```python
from build123d import *

# Parameters (mm, degrees)
CROQUIS1_R              = 1.5
CROQUIS1_R_2            = 4
SALIENTE_EXTRUIR1_DEPTH = 6
CROQUIS4_R              = 4
SALIENTE_EXTRUIR3_DEPTH = 6
CORTAR_EXTRUIR1_DEPTH   = 6
REDONDEO3_R             = 4
CORTAR_EXTRUIR2_DEPTH   = 6
REDONDEO4_R             = 2.5
REDONDEO6_R             = 10


with BuildPart() as part:
    # Croquis1 → Saliente-Extruir1 (new body)
    with BuildSketch(Plane.XY):
        with BuildLine():
            Line((-17.112213819, 2.294275414), (-30.516043414, 23.123582692))
            ThreePointArc((-30.516043414, 23.123582692), (-31.14080226, 23.989156666), (-31.854269143, 24.783201331))
            Line((-31.854269143, 24.783201331), (-45.961940777, 38.890872965))
            Line((-45.961940777, 38.890872965), (-78.488852712, 71.4177849))
            Line((-78.488852712, 71.4177849), (-71.4177849, 78.488852712))
            Line((-71.4177849, 78.488852712), (-38.890872965, 45.961940777))
            Line((-38.890872965, 45.961940777), (-24.783201331, 31.854269143))
            ThreePointArc((-24.783201331, 31.854269143), (-23.989156666, 31.14080226), (-23.123582692, 30.516043414))
            Line((-23.123582692, 30.516043414), (-2.294275414, 17.112213819))
            ThreePointArc((-2.294275414, 17.112213819), (-0.610887166, 15.302496804), (0, 12.907567049))
            Line((0, 12.907567049), (0, 7.055686841))
            ThreePointArc((0, 7.055686841), (-0.823113423, 5.438609853), (-2.614937985, 5.15257064))
            Line((-2.614937985, 5.15257064), (-4.503911831, 5.762938925))
            ThreePointArc((-4.503911831, 5.762938925), (-5.518487605, 5.518487605), (-5.762938925, 4.503911831))
            Line((-5.762938925, 4.503911831), (-5.15257064, 2.614937985))
            ThreePointArc((-5.15257064, 2.614937985), (-5.438609853, 0.823113423), (-7.055686841, 0))
            Line((-7.055686841, 0), (-12.907567049, 0))
            ThreePointArc((-12.907567049, 0), (-15.302496804, 0.610887166), (-17.112213819, 2.294275414))
        make_face()
        with Locations((-38.890872965, 38.890872965)):
            Circle(CROQUIS1_R, mode=Mode.SUBTRACT)
        with Locations((-24.04163056, 24.04163056)):
            Circle(CROQUIS1_R, mode=Mode.SUBTRACT)
        with Locations((-15.25, 15.25)):
            Circle(CROQUIS1_R_2, mode=Mode.SUBTRACT)
    extrude(amount=SALIENTE_EXTRUIR1_DEPTH)

    # Croquis4 → Saliente-Extruir3 (add)
    with BuildSketch(Plane.XY.offset(6)):
        Polygon((-78.488852712, 71.4177849), (-89.802561211, 71.4177849), (-103.944696834, 85.559920524), (-103.944696834, 103.944696834), (-85.559920524, 103.944696834), (-71.4177849, 89.802561211), (-71.4177849, 78.488852712), align=None)
        with Locations((-88.388347648, 88.388347648)):
            Circle(CROQUIS4_R, mode=Mode.SUBTRACT)
    extrude(amount=-SALIENTE_EXTRUIR3_DEPTH)

    # Croquis5 → Cortar-Extruir1 (cut)
    with BuildSketch(Plane.XY.offset(6)):
        with BuildLine():
            Line((-99.348502757, 96.166522241), (-97.227182413, 94.045201898))
            ThreePointArc((-97.227182413, 94.045201898), (-94.045201898, 94.045201898), (-94.045201898, 97.227182413))
            Line((-94.045201898, 97.227182413), (-96.166522241, 99.348502757))
            ThreePointArc((-96.166522241, 99.348502757), (-99.348502757, 99.348502757), (-99.348502757, 96.166522241))
        make_face()
        with BuildLine():
            Line((-89.888347648, 80.638347648), (-89.888347648, 78.638347648))
            ThreePointArc((-89.888347648, 78.638347648), (-88.388347648, 77.138347648), (-86.888347648, 78.638347648))
            Line((-86.888347648, 78.638347648), (-86.888347648, 80.638347648))
            ThreePointArc((-86.888347648, 80.638347648), (-88.388347648, 82.138347648), (-89.888347648, 80.638347648))
        make_face()
        with BuildLine():
            Line((-80.638347648, 86.888347648), (-78.638347648, 86.888347648))
            ThreePointArc((-78.638347648, 86.888347648), (-77.138347648, 88.388347648), (-78.638347648, 89.888347648))
            Line((-78.638347648, 89.888347648), (-80.638347648, 89.888347648))
            ThreePointArc((-80.638347648, 89.888347648), (-82.138347648, 88.388347648), (-80.638347648, 86.888347648))
        make_face()
        with BuildLine():
            Line((-96.138347648, 89.888347648), (-98.138347648, 89.888347648))
            ThreePointArc((-98.138347648, 89.888347648), (-99.638347648, 88.388347648), (-98.138347648, 86.888347648))
            Line((-98.138347648, 86.888347648), (-96.138347648, 86.888347648))
            ThreePointArc((-96.138347648, 86.888347648), (-94.638347648, 88.388347648), (-96.138347648, 89.888347648))
        make_face()
        with BuildLine():
            Line((-86.888347648, 96.138347648), (-86.888347648, 98.138347648))
            ThreePointArc((-86.888347648, 98.138347648), (-88.388347648, 99.638347648), (-89.888347648, 98.138347648))
            Line((-89.888347648, 98.138347648), (-89.888347648, 96.138347648))
            ThreePointArc((-89.888347648, 96.138347648), (-88.388347648, 94.638347648), (-86.888347648, 96.138347648))
        make_face()
    extrude(amount=-CORTAR_EXTRUIR1_DEPTH, mode=Mode.SUBTRACT)

    # Redondeo3
    redondeo3_edges = [part.edges().sort_by_distance(p)[0] for p in [
        (-103.944696834, 103.944696834, 3),
    ]]
    fillet(redondeo3_edges, radius=REDONDEO3_R)

    # Croquis7 → Cortar-Extruir2 (cut)
    with BuildSketch(Plane.XY.offset(6)):
        with BuildLine():
            Line((-103.944696834, 85.559920524), (-89.802561211, 71.4177849))
            ThreePointArc((-89.802561211, 71.4177849), (-95.660425587, 79.702056147), (-103.944696834, 85.559920524))
        make_face()
        with BuildLine():
            Line((-85.559920524, 103.944696834), (-71.4177849, 89.802561211))
            ThreePointArc((-71.4177849, 89.802561211), (-79.702056147, 95.660425587), (-85.559920524, 103.944696834))
        make_face()
    extrude(amount=-CORTAR_EXTRUIR2_DEPTH, mode=Mode.SUBTRACT)

    # Redondeo4
    redondeo4_edges = [part.edges().sort_by_distance(p)[0] for p in [
        (-89.802561211, 71.4177849, 3),
        (-103.944696834, 85.559920524, 3),
        (-85.559920524, 103.944696834, 3),
        (-71.4177849, 89.802561211, 3),
    ]]
    fillet(redondeo4_edges, radius=REDONDEO4_R)

    # Redondeo6
    redondeo6_edges = [part.edges().sort_by_distance(p)[0] for p in [
        (-78.488852712, 71.4177849, 3),
        (-71.4177849, 78.488852712, 3),
    ]]
    fillet(redondeo6_edges, radius=REDONDEO6_R)


solid = part.part
```
Geometry check sheet. Reference: the model listing, model coordinates, mm. A direction names the side the tool comes from. Give positions to 0.01 mm unless a question says otherwise; leave off trailing zeros. Write each loop counter-clockwise with the first axis right and the second up, starting at its lowest first coordinate (ties: lowest second). Pieces come first, ordered by that corner, then holes.
1) Access from +Z, -Z, +X, -X, +Y, -Y to the whole of each face (thin tool, end or side, straight path). Record for faces 1 (the cylindrical face through (-94.64, 88.36, 3.04)), 2 (the cylindrical face through (-15.272, 0.594, 2.958)).
2) Gauge pin test, flat ends, axial feed: pin 1 (7 mm diameter, centred on x = -88.39, y = 88.39, fed in from +Z); pin 2 (3 mm diameter, centred on y = 86.5, z = 4, fed in from +X); pin 3 (1.6 mm diameter, centred on y = 79.5, z = 2.5, fed in from +X); pin 4 (4 mm diameter, centred on x = -24.04, y = 24.04, fed in from -Z). Record the tip position at first contact, or that the pin passes through.
3) Release check for a two-part mould opening along X. For faces 3 (the cylindrical face through (-88.36, 99.64, 3.04)), 4 (the cylindrical face through (-82.14, 88.42, 3.04)), 5 (the flat face through (-56, 56, 6)), 6 (the cylindrical face through (-70.68, 78.86, 3.04)) record: pulls with the +X half, pulls with the -X half, needs draft (parallel to the pull), parting line crosses it, or undercut.
4) Section check C-C, the plane z = 2. State how many separate pieces and enclosed holes the cut face has, and give its area (3 significant figures).
5) Section check D-D, the plane x = -28.5. Record the boundary of the cut face in (y, z), and give its area (3 significant figures).
6) Material ranges on L1, parallel to X at y = 99, z = 3.3; L2, parallel to X at y = 86, z = 3.45; L3, parallel to X at y = 80.5, z = 0.55, recorded low to high.
7) Section check A-A, the plane x = -15.25. Record the boundary of the cut face in (y, z), and give its area (3 significant figures).
8) Section check B-B, the plane y = 15.25. Record the boundary of the cut face in (x, z), and give its area (3 significant figures).
Computed:
1. face 1: +Z, -Z
1. face 2: +Z, -Z, -X, -Y
2. pin 1: passes through
2. pin 2: stops at x = -71.42
2. pin 3: stops at x = -70.61
2. pin 4: stops at z = 0
3. face 3: undercut
3. face 4: undercut
3. face 5: needs draft
3. face 6: pulls with the +X half
4. separate pieces: 1
4. enclosed holes: 9
4. area: 1,800 mm2
5. outline: (19.99, 0) - (35.57, 0) - (35.57, 6) - (19.99, 6) - close
5. area: 93.5 mm2
6. L1: x = -103.94 to -99.63, -95.82 to -89.62, -87.16 to -82.58
6. L2: x = -103.69 to -91.6, -85.18 to -71.42
6. L3: x = -96.49 to -89.89, -86.89 to -71.19
7. outline: (0.58, 0) - (11.25, 0) - (11.25, 6) - (0.58, 6) - close; (19.25, 0) - (25.45, 0) - (25.45, 6) - (19.25, 6) - close
7. area: 101 mm2
8. outline: (-25.45, 0) - (-19.25, 0) - (-19.25, 6) - (-25.45, 6) - close; (-11.25, 0) - (-0.58, 0) - (-0.58, 6) - (-11.25, 6) - close
8. area: 101 mm2
